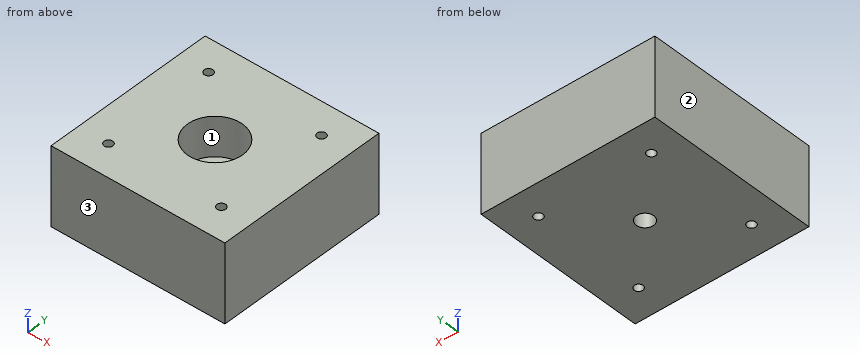
Autodesk Fusion 360 part; units mm, degrees
sketch "Base" plane through (0, 0, 0) normal (0, 0, 1) x (1, 0, 0)
  line L0 (20, 20) -> (-20, 20)
  line L1 (-20, 20) -> (-20, -20)
  line L2 (-20, -20) -> (20, -20)
  line L3 (20, -20) -> (20, 20)
  line L4 (20, 20) -> (-20, -20) construction
  line L5 (-20, 20) -> (20, -20) construction
  circle A0 centre (0, 0) radius 2
  circle A1 centre (0, 0) radius 6.35
  line L6 (13, 13) -> (-13, 13) construction
  line L7 (-13, 13) -> (-13, -13) construction
  line L8 (-13, -13) -> (13, -13) construction
  line L9 (13, -13) -> (13, 13) construction
  line L10 (13, 13) -> (-13, -13) construction
  line L11 (-13, 13) -> (13, -13) construction
  circle A2 centre (-13, 13) radius 1
  circle A3 centre (13, 13) radius 1
  circle A4 centre (13, -13) radius 1
  circle A5 centre (-13, -13) radius 1
  dimension "d1" = 40
  dimension "d2" = 40
  dimension "d3" = 4
  dimension "d6" = 12.7
  dimension "d10" = 26
  dimension "d11" = 26
  dimension "d12" = 2
  dimension "d13" = 2
  dimension "d14" = 2
  dimension "d15" = 2
extrude "Extrude1" add sketch "Base" along normal blind 18 contours L0 L1 L2 L3
extrude "Extrude2" add sketch "Base" along normal blind 9 contours A1
chamfer "Chamfer1" distance 2.5 angle 45 1 edges at (-1.8647, 0.7232, 9)
equation "d13 = d12"
equation "d14 = d12"
equation "d15 = d12"
Check sheet for the modelled part. Datum: model origin and axes. Units: mm. Face numbers are marked on the shaded views. Round coordinates to 2 decimals unless told otherwise and drop trailing zeros. Order: outer loops, then holes, each group sorted by start corner. A loop starts at its lowest first (then second) coordinate and runs counter-clockwise, first axis right, second up.
(1) Cross-section at A-A, the plane y = 0. Enter the section's corners in (x, z).
(2) Go/stop test with a flat-tipped pin: P1, Ø1.8, axis at x = -13, y = -13, coming from the +Z side. Record where the tip stops, or that it passes through.
(3) Cross-section at C-C, the plane x = -13. Enter the section's corners in (y, z), and give its area (3 significant figures).
(4) Scan lines: probe 1 along Y at (x, z) = (13, 7.5); probe 2 along Y at (x, z) = (0, 13.75); probe 3 along Y at (x, z) = (0, 1.5). Record each from-to range of solid material in increasing order.
(5) Draft check along Y on the marked faces 1, 2 and 3. Enter one of: pulls with the +Y half, pulls with the -Y half, needs draft (parallel to the pull), parting line crosses it, or undercut.
(6) Cross-section at B-B, the plane z = 12.25. Enter the section's corners in (x, y), and give its area (3 significant figures).
Check sheet entries:
1. outline: (-20, 0) - (-2, 0) - (-2, 6.5) - (-4.5, 9) - (-6.35, 9) - (-6.35, 18) - (-20, 18) - close; (2, 0) - (20, 0) - (20, 18) - (6.35, 18) - (6.35, 9) - (4.5, 9) - (2, 6.5) - close
2. P1: passes through
3. outline: (-20, 0) - (-14, 0) - (-14, 18) - (-20, 18) - close; (-12, 0) - (12, 0) - (12, 18) - (-12, 18) - close; (14, 0) - (20, 0) - (20, 18) - (14, 18) - close
3. area: 648 mm2
4. probe 1: y = -20 to -14, -12 to 12, 14 to 20
4. probe 2: y = -20 to -6.35, 6.35 to 20
4. probe 3: y = -20 to -2, 2 to 20
5. face 1: undercut
5. face 2: needs draft
5. face 3: pulls with the -Y half
6. outline: (-20, -20) - (20, -20) - (20, 20) - (-20, 20) - close; hole circle Ø2 at (-13, -13); hole circle Ø2 at (-13, 13); hole circle Ø12.7 at (0, 0); hole circle Ø2 at (13, -13); hole circle Ø2 at (13, 13)
6. area: 1,460 mm2
